```python
from build123d import *

# Parameters (mm, degrees)
F1_DEPTH = 9.144
F3_DEPTH = 25.4
F4_R     = 5.499555
F5_DEPTH = 43.892203


with BuildPart() as f1:
    # F0 (on Front) → F1 (new body)
    with BuildSketch(Plane.XZ):
        Polygon((0, 34.29), (0, 0), (43.891203, 0), (26.5176, 34.29), align=None)
    extrude(amount=-F1_DEPTH)

    # F2 (on Front) → F3 (join)
    with BuildSketch(Plane.XZ):
        Polygon((38.196363, 0), (23.010547, 29.972), (0, 29.972), (0, 0), align=None)
    extrude(amount=F3_DEPTH)

    # F4 (on face) → F5 (cut, through all)
    with BuildSketch(Plane(origin=(0, 0, 0), x_dir=(0, -1, 0), z_dir=(-1, 0, 0))):
        with Locations((12.7, 14.986)):
            Circle(F4_R)
    extrude(amount=-F5_DEPTH, mode=Mode.SUBTRACT)


solid = f1.part
```
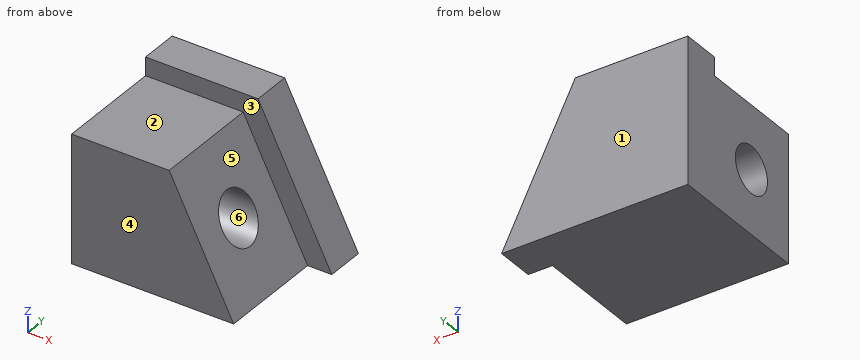
Part model, mm, in its own coordinate system. Face numbers are marked on the shaded views. A direction names the side the tool comes from. Give positions to 0.01 mm unless a question says otherwise; leave off trailing zeros. Order: outer loops, then holes, each group sorted by start corner. A loop starts at its lowest first (then second) coordinate and runs counter-clockwise, first axis right, second up. Notation, with made-up numbers: (87, -4.75) - (99, -4.75) arc R13 cw to (99, 13.25) - close; hole circle Ø2 at (1, 58). An arc over 180 degrees is marked (long way). Use one line per item in the form item = value.
Item 1: Slice it at A-A on y = -12.7. Give the cut face in (x, z).
Solution:
outline = (0, 0) - (38.2, 0) - (33.39, 9.49) - (0, 9.49) - close; (0, 20.49) - (27.82, 20.49) - (23.01, 29.97) - (0, 29.97) - close
Item 2: Slice it at B-B on z = 12. Give the cut face in (x, y).
Solution:
outline = (0, -25.4) - (32.12, -25.4) - (32.12, -17.32) - (0, -17.32) - close; (0, -8.08) - (32.12, -8.08) - (32.12, 0) - (37.81, 0) - (37.81, 9.14) - (0, 9.14) - close
Item 3: Pin check, flat tips, straight feed: pin 1 Ø12 at (y, z) = (-12, 9) entering from +X; pin 2 Ø4 at (y, z) = (2, 9) entering from +X; pin 3 Ø4 at (x, z) = (37, 17.5) entering from +Y; pin 4 Ø8 at (x, z) = (38.5, 10.5) entering from -Y. Stop position of each tip, or through.
Solution:
pin_1 = 36.68
pin_2 = 40.34
pin_3 = 9.14
pin_4 = 0
Item 4: Probe probe 1 along Z at (x, y) = (8.5, -12.7); probe 2 along Y at (x, z) = (13, 31); probe 3 along Z at (x, y) = (7, -12). List the from-to ranges inside material, lowest first. Write a range as from..to.
Solution:
probe_1 = 0..9.49, 20.49..29.97
probe_2 = 0..9.14
probe_3 = 0..9.53, 20.44..29.97
Item 5: Which spindle directions (+Z, -Z, +X, -X, +Y, -Y) get a long thin tool onto all of the face, cutting with end or side? Do the marked faces 1, 2 and 3. Say none if no direction does.
Solution:
face_1 = +Z, -Z, +X, -X, +Y
face_2 = +Z, +X, -X, -Y
face_3 = +Z, +X, -Y
Item 6: Slice it at D-D on x = 20. Give the cut face in (y, z).
Solution:
outline = (-25.4, 0) - (9.14, 0) - (9.14, 34.29) - (0, 34.29) - (0, 29.97) - (-25.4, 29.97) - close; hole circle Ø11 at (-12.7, 14.99)
Item 7: Slice it at C-C on x = 40. Give the cut face in (y, z), and give its area (3 significant figures).
Solution:
outline = (0, 0) - (9.14, 0) - (9.14, 7.68) - (0, 7.68) - close
area = 70.2 mm2
Item 8: Two-plate mould, pull along Y, no slides. Class the marked faces 4, 5 and 6: released by +Y, released by -Y, zero draft, split by the parting line, or undercut.
Solution:
face_4 = released by -Y
face_5 = zero draft
face_6 = undercut
